```python
from build123d import *

# Parameters (mm, degrees)
SKETCH1_W             = 50
SKETCH1_H             = 44
BOSS_EXTRUDE1_DEPTH   = 6.5
SKETCH2_W             = 38
SKETCH2_H             = 7
CUT_EXTRUDE1_DEPTH    = 56.011362463
F_8_0MM_DOWEL_HOLE1_D = 8
CHAMFER1_SIZE         = 3


with BuildPart() as part:
    # Sketch1 → Boss-Extrude1 (new, symmetric)
    with BuildSketch(Plane(origin=(0, 0, 0), x_dir=(1, 0, 0), z_dir=(0, 1, 0))):
        Rectangle(SKETCH1_W, SKETCH1_H)
    extrude(amount=BOSS_EXTRUDE1_DEPTH, both=True)

    # Sketch2 → Cut-Extrude1 (cut, through all)
    with BuildSketch(Plane(origin=(25, 0, 0), x_dir=(0, 0, -1), z_dir=(1, 0, 0))):
        with Locations((3, 3)):
            Rectangle(SKETCH2_W, SKETCH2_H)
    extrude(amount=-CUT_EXTRUDE1_DEPTH, mode=Mode.SUBTRACT)

    # Ø8.0mm Dowel Hole1 (through all)
    with Locations(Plane(origin=(0, -6.5, 0), x_dir=(-1, 0, 0), z_dir=(0, -1, 0))):
        with Locations((0, 14), (0, -4)):
            Hole(F_8_0MM_DOWEL_HOLE1_D / 2)

    # Chamfer1
    chamfer1_edges = [part.edges().sort_by_distance(p)[0] for p in [
        (-4, -6.5, 4),
        (-4, -6.5, -14),
    ]]
    chamfer(chamfer1_edges, length=CHAMFER1_SIZE)


solid = part.part
```
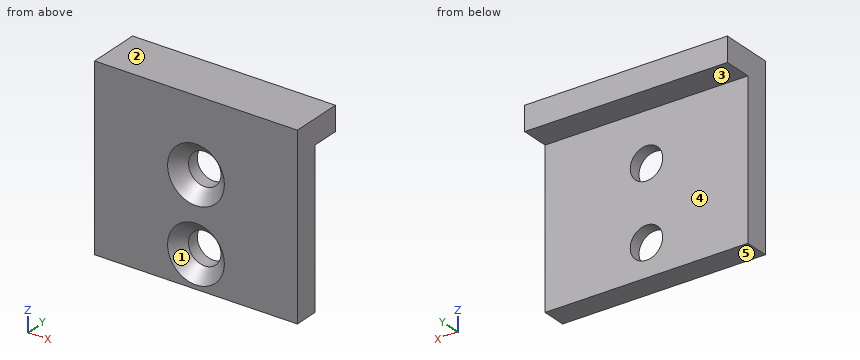
Model file for the job. Use its own axes, mm. Face numbers are marked on the shaded views. A direction names the side the tool comes from. Coordinates: 2 decimals unless noted, no trailing zeros. Order: outer loops, then holes, each group sorted by start corner. A loop starts at its lowest first (then second) coordinate and runs counter-clockwise, first axis right, second up. Notation, with made-up numbers: (65.5, 21) - (100.5, 21) arc R11 ccw to (100.5, 36) - close; hole circle Ø5 at (49.25, -33). An arc over 180 degrees is marked (long way). Return JSON: item names as keys, results as strings. Group by question number.
1) Flat gauge pins, fed straight in: P1, Ø13, axis at x = 0, z = -14, coming from the -Y side; P2, Ø5, axis at x = -0.5, y = 3, coming from the -Z side; P3, Ø6, axis at x = -3.5, z = 1, coming from the +Y side; P4, Ø7, axis at x = 0, z = 4, coming from the +Y side. Where does each tip first touch, or does it go through?
2) Saw through at C-C, the plane x = 0. Write the cut outline in (y, z).
3) Probe line 1 (Z direction, x = 0, y = -1.3); line 2 (X direction, y = -1.3, z = 4); line 3 (Z direction, x = -15, y = 5.5). List the from-to ranges inside material, lowest first. Write a range as from..to.
4) Mould opens along Z. For the marked faces 1, 2 and 3 say: released by +Z, released by -Z, zero draft, split by the parting line, or undercut.
5) Saw through at B-B, the plane y = -1.75. Write the cut outline in (x, z), plus the area to 3 significant figures.
6) Tool access for the marked faces 4 and 5: list every direction of +Z, -Z, +X, -X, +Y, -Y with a clear straight run to the whole face (end or side of a thin tool).
7) Saw through at D-D, the plane x = 10.5. Write the cut outline in (y, z), plus the area to 3 significant figures.
8) Saw through at A-A, the plane z = 4. Write the cut outline in (x, y).
Values found:
{
 "1": {"P1": "stops at y = -6", "P2": "stops at z = 16", "P3": "stops at y = -0.5", "P4": "passes through"},
 "2": {"outline": "(-6.5, -22) - (-0.5, -22) - (-0.5, -18) - (-3.5, -18) - (-6.5, -21) - close; (-6.5, -7) - (-3.5, -10) - (-0.5, -10) - (-0.5, 0) - (-3.5, 0) - (-6.5, -3) - close; (-6.5, 11) - (-3.5, 8) - (-0.5, 8) - (-0.5, 16) - (6.5, 16) - (6.5, 22) - (-6.5, 22) - close"},
 "3": {"line 1": "z = -22..-18, -10..0, 8..22", "line 2": "x = -25..-4, 4..25", "line 3": "z = 16..22"},
 "4": {"face 1": "undercut", "face 2": "released by +Z", "face 3": "released by -Z"},
 "5": {"outline": "(-25, -22) - (25, -22) - (25, 22) - (-25, 22) - close; hole circle Ø8 at (0, -14); hole circle Ø8 at (0, 4)", "area": "2,100 mm²"},
 "6": {"face 4": "-Z, +X, -X, +Y", "face 5": "-Z, +X, -X, +Y, -Y"},
 "7": {"outline": "(-6.5, -22) - (-0.5, -22) - (-0.5, 16) - (6.5, 16) - (6.5, 22) - (-6.5, 22) - close", "area": "306 mm²"},
 "8": {"outline": "(-25, -6.5) - (-7, -6.5) - (-4, -3.5) - (-4, -0.5) - (-25, -0.5) - close; (4, -3.5) - (7, -6.5) - (25, -6.5) - (25, -0.5) - (4, -0.5) - close"}
}
